from build123d import *

# Parameters (mm, degrees)
SKETCH1_R           = 18
SKETCH1_R_2         = 6
BOSS_EXTRUDE4_DEPTH = 8
SKETCH5_R           = 20
SKETCH5_R_2         = 15.5
BOSS_EXTRUDE5_DEPTH = 3
SKETCH6_W           = 34
SKETCH6_H           = 4
BOSS_EXTRUDE6_DEPTH = 57
CUT_EXTRUDE1_REACH  = 139.135
CUT_EXTRUDE2_REACH  = 139.135
SKETCH9_R           = 2
BOSS_EXTRUDE8_DEPTH = 3
FILLET1_R           = 10
FILLET2_R           = 10


with BuildPart() as part:
    # Sketch1 → Boss-Extrude4 (new body)
    with BuildSketch(Plane(origin=(0, 0, 0), x_dir=(1, 0, 0), z_dir=(0, 1, 0))):
        with BuildLine():
            Line((0, 0), (-32.22015265, -19.667505907))
            ThreePointArc((-32.22015265, -19.667505907), (-39.781284933, -38.449706153), (-27.069479945, -54.208887014))
            Line((-27.069479945, -54.208887014), (0, -71))
            Line((0, -71), (111, -71))
            Line((111, -71), (111, 0))
            Line((111, 0), (0, 0))
        make_face()
        with Locations(Location((35.5, -35.5, 0), (0, 0, 270))):
            Circle(SKETCH1_R, mode=Mode.SUBTRACT)
        with Locations(Location((-20, -35.5, 0), (0, 0, 270))):
            Circle(SKETCH1_R_2, mode=Mode.SUBTRACT)
    extrude(amount=BOSS_EXTRUDE4_DEPTH)

    # Sketch5 → Boss-Extrude5 (add)
    with BuildSketch(Plane(origin=(0, 8, 0), x_dir=(1, 0, 0), z_dir=(0, 1, 0))):
        with Locations(Location((-20, -35.5, 0), (0, 0, 115.138226689))):
            Circle(SKETCH5_R)
        with Locations(Location((-20, -35.5, 0), (0, 0, 270))):
            Circle(SKETCH5_R_2, mode=Mode.SUBTRACT)
    extrude(amount=BOSS_EXTRUDE5_DEPTH)

    # Sketch6 → Boss-Extrude6 (add)
    with BuildSketch(Plane(origin=(111, 0, 0), x_dir=(0, 0, -1), z_dir=(1, 0, 0))):
        Polygon((-71, 38), (-71, 8), (-67, 8), (-67, 34), (-67, 38), align=None)
        with Locations((-50, 36)):
            Rectangle(SKETCH6_W, SKETCH6_H)
        Polygon((-33, 34), (-33, 8), (-29, 8), (-29, 38), (-33, 38), align=None)
    extrude(amount=-BOSS_EXTRUDE6_DEPTH)

    # Sketch7 → Cut-Extrude1 (cut, up to next)
    with BuildSketch(Plane(origin=(0, 38, 0), x_dir=(1, 0, 0), z_dir=(0, 1, 0)), mode=Mode.PRIVATE) as cut_extrude1_sk1:
        with BuildLine():
            Line((74, -45.5), (54, -45.5))
            Line((54, -45.5), (54, -50))
            Line((54, -50), (54, -54.5))
            Line((54, -54.5), (74, -54.5))
            ThreePointArc((74, -54.5), (78.5, -50), (74, -45.5))
        make_face()
    cut_extrude1_tool1 = extrude(cut_extrude1_sk1.sketch, amount=-CUT_EXTRUDE1_REACH, mode=Mode.PRIVATE) & part.part
    # Sketch7 → Cut-Extrude1 (cut, up to next)
    with BuildSketch(Plane(origin=(0, 38, 0), x_dir=(1, 0, 0), z_dir=(0, 1, 0)), mode=Mode.PRIVATE) as cut_extrude1_sk2:
        with BuildLine():
            Line((60, -57.5), (66, -57.5))
            ThreePointArc((66, -57.5), (67.5, -59), (66, -60.5))
            Line((66, -60.5), (60, -60.5))
            ThreePointArc((60, -60.5), (58.5, -59), (60, -57.5))
        make_face()
    cut_extrude1_tool2 = extrude(cut_extrude1_sk2.sketch, amount=-CUT_EXTRUDE1_REACH, mode=Mode.PRIVATE) & part.part
    # Sketch7 → Cut-Extrude1 (cut, up to next)
    with BuildSketch(Plane(origin=(0, 38, 0), x_dir=(1, 0, 0), z_dir=(0, 1, 0)), mode=Mode.PRIVATE) as cut_extrude1_sk3:
        with BuildLine():
            Line((60, -39.5), (66, -39.5))
            ThreePointArc((66, -39.5), (67.5, -41), (66, -42.5))
            Line((66, -42.5), (60, -42.5))
            ThreePointArc((60, -42.5), (58.5, -41), (60, -39.5))
        make_face()
    cut_extrude1_tool3 = extrude(cut_extrude1_sk3.sketch, amount=-CUT_EXTRUDE1_REACH, mode=Mode.PRIVATE) & part.part
    # Sketch7 → Cut-Extrude1 (cut, up to next)
    with BuildSketch(Plane(origin=(0, 38, 0), x_dir=(1, 0, 0), z_dir=(0, 1, 0)), mode=Mode.PRIVATE) as cut_extrude1_sk4:
        with BuildLine():
            Line((93, -57.5), (99, -57.5))
            ThreePointArc((99, -57.5), (100.5, -59), (99, -60.5))
            Line((99, -60.5), (93, -60.5))
            ThreePointArc((93, -60.5), (91.5, -59), (93, -57.5))
        make_face()
    cut_extrude1_tool4 = extrude(cut_extrude1_sk4.sketch, amount=-CUT_EXTRUDE1_REACH, mode=Mode.PRIVATE) & part.part
    # Sketch7 → Cut-Extrude1 (cut, up to next)
    with BuildSketch(Plane(origin=(0, 38, 0), x_dir=(1, 0, 0), z_dir=(0, 1, 0)), mode=Mode.PRIVATE) as cut_extrude1_sk5:
        with BuildLine():
            Line((93, -42.5), (99, -42.5))
            ThreePointArc((99, -42.5), (100.5, -41), (99, -39.5))
            Line((99, -39.5), (93, -39.5))
            ThreePointArc((93, -39.5), (91.5, -41), (93, -42.5))
        make_face()
    cut_extrude1_tool5 = extrude(cut_extrude1_sk5.sketch, amount=-CUT_EXTRUDE1_REACH, mode=Mode.PRIVATE) & part.part
    add(cut_extrude1_tool1.solids().sort_by_distance((65.788578, 38, 50))[0], mode=Mode.SUBTRACT)
    add(cut_extrude1_tool2.solids().sort_by_distance((63, 38, 59))[0], mode=Mode.SUBTRACT)
    add(cut_extrude1_tool3.solids().sort_by_distance((63, 38, 41))[0], mode=Mode.SUBTRACT)
    add(cut_extrude1_tool4.solids().sort_by_distance((96, 38, 59))[0], mode=Mode.SUBTRACT)
    add(cut_extrude1_tool5.solids().sort_by_distance((96, 38, 41))[0], mode=Mode.SUBTRACT)

    # Sketch9 → Cut-Extrude2 (cut, up to next)
    with BuildSketch(Plane.XZ, mode=Mode.PRIVATE) as cut_extrude2_sk1:
        with Locations(Location((64.5, 64.5, 0), (0, 0, 270))):
            Circle(SKETCH9_R)
    cut_extrude2_tool1 = extrude(cut_extrude2_sk1.sketch, amount=-CUT_EXTRUDE2_REACH, mode=Mode.PRIVATE) & part.part
    # Sketch9 → Cut-Extrude2 (cut, up to next)
    with BuildSketch(Plane.XZ, mode=Mode.PRIVATE) as cut_extrude2_sk2:
        with Locations(Location((6.5, 64.5, 0), (0, 0, 270))):
            Circle(SKETCH9_R)
    cut_extrude2_tool2 = extrude(cut_extrude2_sk2.sketch, amount=-CUT_EXTRUDE2_REACH, mode=Mode.PRIVATE) & part.part
    # Sketch9 → Cut-Extrude2 (cut, up to next)
    with BuildSketch(Plane.XZ, mode=Mode.PRIVATE) as cut_extrude2_sk3:
        with Locations(Location((6.5, 6.5, 0), (0, 0, 270))):
            Circle(SKETCH9_R)
    cut_extrude2_tool3 = extrude(cut_extrude2_sk3.sketch, amount=-CUT_EXTRUDE2_REACH, mode=Mode.PRIVATE) & part.part
    # Sketch9 → Cut-Extrude2 (cut, up to next)
    with BuildSketch(Plane.XZ, mode=Mode.PRIVATE) as cut_extrude2_sk4:
        with Locations(Location((64.5, 6.5, 0), (0, 0, 270))):
            Circle(SKETCH9_R)
    cut_extrude2_tool4 = extrude(cut_extrude2_sk4.sketch, amount=-CUT_EXTRUDE2_REACH, mode=Mode.PRIVATE) & part.part
    add(cut_extrude2_tool1.solids().sort_by_distance((64.5, 0, 64.5))[0], mode=Mode.SUBTRACT)
    add(cut_extrude2_tool2.solids().sort_by_distance((6.5, 0, 64.5))[0], mode=Mode.SUBTRACT)
    add(cut_extrude2_tool3.solids().sort_by_distance((6.5, 0, 6.5))[0], mode=Mode.SUBTRACT)
    add(cut_extrude2_tool4.solids().sort_by_distance((64.5, 0, 6.5))[0], mode=Mode.SUBTRACT)

    # Sketch10 → Boss-Extrude8 (add)
    with BuildSketch(Plane(origin=(0, 8, 0), x_dir=(1, 0, 0), z_dir=(0, 1, 0))):
        with BuildLine():
            Line((17.5, -15.5), (-20, -15.5))
            ThreePointArc((-20, -15.5), (-5.857864376, -21.357864376), (0, -35.5))
            ThreePointArc((0, -35.5), (-5.857864376, -49.642135624), (-20, -55.5))
            Line((-20, -55.5), (17.5, -55.5))
            Line((17.5, -55.5), (17.5, -15.5))
        make_face()
    extrude(amount=BOSS_EXTRUDE8_DEPTH)

    # Fillet1
    # the kernel refuses this fillet: 10 mm, written as the material it takes off along each edge
    with BuildSketch(Plane(origin=(111, 63, 71), x_dir=(-1, 0, 0), z_dir=(0, -1, 0))) as fillet1_piece_1:
        with BuildLine():
            CenterArc((FILLET1_R, FILLET1_R), FILLET1_R, 180, 90)
            Line((0, FILLET1_R), (0, 0))
            Line((0, 0), (FILLET1_R, 0))
        make_face()
    extrude(amount=88, mode=Mode.SUBTRACT)

    # Fillet2
    fillet2_edges = [part.edges().sort_by_distance(p)[0] for p in [
        (111, 4, 0),
    ]]
    fillet(fillet2_edges, radius=FILLET2_R)


solid = part.part
The listing builds one solid part. Answer for the finished solid, in the listing's coordinates (mm). A direction names the side the tool comes from. Coordinates: 2 decimals unless noted, no trailing zeros. Loops run counter-clockwise (first coordinate to the right, second up) from the corner with the lowest first, then second, coordinate; pieces in that order, holes last.
1) Determine the mould class of faces 1 (the face through (67.5, 36, 41)), 2 (the face through (-13.7, 3.9, 62.5)), 3 (the face through (1, 11, 35)) for opening direction Z: pulls with the +Z half, pulls with the -Z half, needs draft (parallel to the pull), parting line crosses it, or undercut.
2) Flat-ended cylindrical pins translate along their axes: pin 1 Ø6 at (y, z) = (28.5, 44.5) entering from -X (3 decimals); pin 2 Ø2 at (x, y) = (60, 36) entering from -Z; pin 3 Ø13 at (y, z) = (18.5, 66) entering from -X; pin 4 Ø3.5 at (x, y) = (-4.5, 9) entering from -Z. Find the tip coordinate at first contact, or state that the pin passes through.
3) A tool of negligible diameter and unlimited length cuts with its end or side. For faces 4 (the face through (64, 36, 45.5)), 5 (the face through (83, 38, 50)), 6 (the face through (-13, 8, 35)), from which of +Z, -Z, +X, -X, +Y, -Y can it reach the whole face along a straight path? Write none if from no direction.
4) Find the intervals of material crossed by L1, parallel to X at y = 5, z = 35; L2, parallel to Z at x = 6, y = 4; L3, parallel to Z at x = 69, y = 19.5, in increasing order.
5) Find section D-D on x = 85. Write down the section's boundary in (y, z).
6) Find section C-C on y = 21. Write down the section's boundary in (x, z).
7) Find section A-A on x = 35.5. Write down the section's boundary in (y, z).
8) Find section B-B on x = 6.5. Write down the section's boundary in (y, z), then the cut area to 3 significant figures.
Values:
1. face 1: undercut
1. face 2: pulls with the +Z half
1. face 3: needs draft
2. pin 1: passes through
2. pin 2: stops at z = 29
2. pin 3: stops at x = 54
2. pin 4: stops at z = 1.87
3. face 4: -X, +Y
3. face 5: +Z, -Z, +X, -X, +Y
3. face 6: +Y
4. L1: x = -39.99 to -25.98, -14.02 to 17.51, 53.49 to 111
4. L2: z = 0 to 4.56, 8.44 to 62.56, 66.44 to 71
4. L3: z = 29 to 33, 67 to 71
5. outline: (0, 0) - (8, 0) - (8, 29) - (38, 29) - (38, 71) - (0, 71) - close; hole (8, 33) - (34, 33) - (34, 67) - (8, 67) - close
6. outline: (54, 29) - (111, 29) - (111, 33) - (54, 33) - close; (54, 67) - (109, 67) arc R10 ccw to (101, 71) - (54, 71) - close
7. outline: (0, 0) - (8, 0) - (8, 17.5) - (0, 17.5) - close; (0, 53.5) - (8, 53.5) - (8, 71) - (0, 71) - close
8. outline: (0, 0) - (8, 0) - (8, 4.5) - (0, 4.5) - close; (0, 8.5) - (8, 8.5) - (8, 15.5) - (11, 15.5) - (11, 55.5) - (8, 55.5) - (8, 62.5) - (0, 62.5) - close; (0, 66.5) - (8, 66.5) - (8, 71) - (0, 71) - close
8. area: 624 mm2
